```python
from build123d import *

# Parameters (mm, degrees)
BOSS_EXTRUDE3_DEPTH        = 10
SKETCH4_R                  = 1.5
BOSS_EXTRUDE4_DEPTH        = 5
RIB6_REACH                 = 158.985
SKETCH5_WALL_W             = 329.861950248
SKETCH5_WALL_H             = 2.5
CHAMFER2_SIZE              = 1
LPATTERN4_COUNT            = 2
LPATTERN4_PITCH            = 75
LPATTERN4_COPY_1_REACH     = 158.985
LPATTERN4_COPY_1_SKETCH_W  = 329.861950248
LPATTERN4_COPY_1_SKETCH_H  = 2.5
CHAMFER2_OF_LPATTERN4_SIZE = 1
CHAMFER3_SIZE              = 9
SKETCH8_R                  = 2.05
CUT_EXTRUDE1_DEPTH         = 4
SKETCH9_R                  = 1.6
CUT_EXTRUDE2_DEPTH         = 5


with BuildPart() as part:
    # Sketch2 → Boss-Extrude3 (new body)
    with BuildSketch(Plane(origin=(0, 0, 0), x_dir=(1, 0, 0), z_dir=(0, 1, 0))):
        with BuildLine():
            Line((-138.973021921, 39.179223473), (-139.052157616, 4.179312937))
            Line((-139.052157616, 4.179312937), (73.947297933, 3.697715709))
            Line((73.947297933, 3.697715709), (74.026978079, 38.697625014))
            Line((74.026978079, 38.697625014), (67.526578048, 38.712322585))
            Line((67.526578048, 38.712322585), (67.51414235, 33.212297518))
            Line((67.51414235, 33.212297518), (58.599731895, 33.232453229))
            ThreePointArc((58.599731895, 33.232453229), (42.488076808, 21.768891824), (26.428425, 33.305193378))
            Line((26.428425, 33.305193378), (17.51414235, 33.3253488))
            Line((17.51414235, 33.3253488), (17.526578048, 38.825373866))
            Line((17.526578048, 38.825373866), (-7.473230244, 38.881899074))
            Line((-7.473230244, 38.881899074), (-7.485665941, 33.381874007))
            Line((-7.485665941, 33.381874007), (-16.400076396, 33.402029717))
            ThreePointArc((-16.400076396, 33.402029717), (-32.511731484, 21.938468313), (-48.571383292, 33.474769867))
            Line((-48.571383292, 33.474769867), (-57.485665941, 33.494925288))
            Line((-57.485665941, 33.494925288), (-57.473230244, 38.994950355))
            Line((-57.473230244, 38.994950355), (-82.473038536, 39.051475562))
            Line((-82.473038536, 39.051475562), (-82.485474233, 33.551450496))
            Line((-82.485474233, 33.551450496), (-91.399884688, 33.571606206))
            ThreePointArc((-91.399884688, 33.571606206), (-107.511539776, 22.108044802), (-123.571191584, 33.644346356))
            Line((-123.571191584, 33.644346356), (-132.485474233, 33.664501777))
            Line((-132.485474233, 33.664501777), (-132.473038536, 39.164526844))
            Line((-132.473038536, 39.164526844), (-138.973021921, 39.179223473))
        make_face()
    extrude(amount=BOSS_EXTRUDE3_DEPTH)

    # Sketch4 → Boss-Extrude4 (add)
    with BuildSketch(Plane(origin=(0.087874316, 0, -38.864803222), x_dir=(-0.99999744389135, 0, -0.002261019850970016), z_dir=(0.002261019850970016, 0, -0.99999744389135))):
        Polygon((62.56118779, -12), (57.561251693, 0), (82.561123887, 0), (77.56118779, -12), align=None)
        with Locations((70.06118779, -8.5)):
            Circle(SKETCH4_R, mode=Mode.SUBTRACT)
    boss_extrude4 = extrude(amount=-BOSS_EXTRUDE4_DEPTH)

    # Sketch5 wall → Rib6 (add, up to next)
    with BuildSketch(Plane(origin=(-77.492333887, -6, -30.540192335), x_dir=(-0.001139262394, 0.863778900906, 0.503869737562), z_dir=(-0.001953021242, -0.503871025511, 0.863776692993)), mode=Mode.PRIVATE) as rib6_sk1:
        with Locations((0, -1.25)):
            Rectangle(SKETCH5_WALL_W, SKETCH5_WALL_H)
    rib6_tool1 = extrude(rib6_sk1.sketch, amount=-RIB6_REACH, mode=Mode.PRIVATE) - part.part
    rib6 = rib6_tool1.solids().sort_by_distance((-77.492333887, -6, -30.540192335))[0]
    add(rib6)

    # Mirror2: Rib6 across plane
    add(rib6.mirror(Plane(origin=(-70.061008706, 0, -0.158409736), x_dir=(-0.0022610198509701073, 0, 0.99999744389135), z_dir=(0.99999744389135, 0, 0.002261019850970107))))

    # Chamfer2
    chamfer2_edges = [part.edges().sort_by_distance(p)[0] for p in [
        (-68.484443323, -8.5, -34.01983421),
    ]]
    chamfer(chamfer2_edges, length=CHAMFER2_SIZE)

    # LPattern4: Boss-Extrude4, Rib6 ×2
    with Locations(*[Vector(0.9999974438913499, 0, 0.002261019850970079) * (i * LPATTERN4_PITCH) for i in range(1, LPATTERN4_COUNT)]):
        add(boss_extrude4)
        add(rib6)

    # LPattern4 copy 1 sketch → LPattern4 copy 1 (add, up to next)
    with BuildSketch(Plane(origin=(12.507436062, -6, -30.336700548), x_dir=(-0.0011392623880184954, 0.863778900906, 0.5038697375620136), z_dir=(-0.0019530212415939509, -0.503871025511, 0.863776692993001)), mode=Mode.PRIVATE) as lpattern4_copy_1_sk1:
        with Locations((0, 1.25)):
            Rectangle(LPATTERN4_COPY_1_SKETCH_W, LPATTERN4_COPY_1_SKETCH_H)
    lpattern4_copy_1_tool1 = extrude(lpattern4_copy_1_sk1.sketch, amount=-LPATTERN4_COPY_1_REACH, mode=Mode.PRIVATE) - part.part
    add(lpattern4_copy_1_tool1.solids().sort_by_distance((12.507436062, -6, -30.336700548))[0])

    # Chamfer2 of LPattern4
    chamfer2_of_lpattern4_edges = [part.edges().sort_by_distance(p)[0] for p in [
        (6.515364969, -8.5, -33.850257721),
    ]]
    chamfer(chamfer2_of_lpattern4_edges, length=CHAMFER2_OF_LPATTERN4_SIZE)

    # Chamfer3
    chamfer3_edges = [part.edges().sort_by_distance(p)[0] for p in [
        (-32.552429841, 0, -3.938514323),
    ]]
    chamfer(chamfer3_edges, length=CHAMFER3_SIZE)

    # Sketch8 → Cut-Extrude1 (cut)
    with BuildSketch(Plane(origin=(0, 10, 0), x_dir=(1, 0, 0), z_dir=(0, 1, 0))):
        with Locations(Location((-129.018242433, 19.156613217, 0), (0, 0, 270))):
            Circle(SKETCH8_R)
    cut_extrude1 = extrude(amount=-CUT_EXTRUDE1_DEPTH, mode=Mode.SUBTRACT)

    # Sketch9 → Cut-Extrude2 (cut)
    with BuildSketch(Plane(origin=(0, 6, 0), x_dir=(1, 0, 0), z_dir=(0, 1, 0))):
        with Locations(Location((-129.018242433, 19.156613217, 0), (0, 0, 270))):
            Circle(SKETCH9_R)
    cut_extrude2 = extrude(amount=-CUT_EXTRUDE2_DEPTH, mode=Mode.SUBTRACT)

    # Mirror4: Cut-Extrude1, Cut-Extrude2 across plane
    add(cut_extrude1.mirror(Plane(origin=(-32.561168463, 0, -0.073621636), x_dir=(-0.002261019850969509, 0, 0.99999744389135), z_dir=(-0.99999744389135, 0, -0.0022610198509695084))), mode=Mode.SUBTRACT)
    add(cut_extrude2.mirror(Plane(origin=(-32.561168463, 0, -0.073621636), x_dir=(-0.002261019850969509, 0, 0.99999744389135), z_dir=(-0.99999744389135, 0, -0.0022610198509695084))), mode=Mode.SUBTRACT)


solid = part.part
```
Check sheet for the modelled part. Datum: model origin and axes. Units: mm. A direction names the side the tool comes from. Round coordinates to 2 decimals unless told otherwise and drop trailing zeros. Order: outer loops, then holes, each group sorted by start corner. A loop starts at its lowest first (then second) coordinate and runs counter-clockwise, first axis right, second up.
1) Section check B-B (y = 3). Record the boundary of the cut face in (x, z).
2) Go/stop test with flat-tipped pins: pin 1 Ø2 at (x, z) = (-8.5, -26) entering from -Y; pin 2 Ø12 at (x, y) = (11.5, 6) entering from -Z; pin 3 Ø2 at (x, z) = (63, -18.5) entering from +Y. Record where each tip stops, or that it passes through.
3) Section check A-A (z = -29). Give the number of separate pieces and of enclosed holes in the cut face, and give its area (3 significant figures).
4) Section check C-C (x = -104). Record the boundary of the cut face in (y, z).
5) Scan lines: line 1 (X direction, y = -1.25, z = -28.5); line 2 (X direction, y = 0.75, z = -35); line 3 (Z direction, x = -53, y = 0.25). Record each from-to range of solid material in increasing order.
6) Section check D-D (x = -39). Record the boundary of the cut face in (y, z).
7) Tool access check on faces 1 (the cylindrical face through (-107.22, 4.93, -22.11)), 2 (the flat face through (-34, 0, -20)). Record the directions out of +Z, -Z, +X, -X, +Y, -Y that give a thin tool (end or side, any length) a straight path to the whole face; none if there is none.
Result:
1. outline: (-139.04, -10.18) - (-138.97, -39.18) - (-132.47, -39.16) - (-132.49, -33.66) - (-123.57, -33.64) arc R17 cw to (-91.4, -33.57) - (-82.49, -33.55) - (-82.47, -39.05) - (-57.47, -38.99) - (-57.49, -33.49) - (-48.57, -33.47) arc R17 cw to (-16.4, -33.4) - (-7.49, -33.38) - (-7.47, -38.88) - (17.53, -38.83) - (17.51, -33.33) - (26.43, -33.31) arc R17 cw to (58.6, -33.23) - (67.51, -33.21) - (67.53, -38.71) - (74.03, -38.7) - (73.96, -9.7) - close; hole circle Ø3.2 at (-129.02, -19.16); hole circle Ø3.2 at (63.98, -18.72)
2. pin 1: stops at y = 0
2. pin 2: stops at z = -38.85
2. pin 3: stops at y = 6
3. separate pieces: 4
3. enclosed holes: 0
3. area: 1,340 mm2
4. outline: (0, -22.47) - (10, -22.47) - (10, -4.1) - (9, -4.1) - (0, -13.1) - close
5. line 1: x = -77.5 to -75, -65 to -62.5, -2.5 to 0, 10 to 12.5
5. line 2: x = -138.98 to -132.48, -82.48 to -57.48, -7.48 to 17.52, 67.52 to 74.02
5. line 3: z = -33.48 to -12.73
6. outline: (0, -23.24) - (10, -23.24) - (10, -3.95) - (9, -3.95) - (0, -12.95) - close
7. face 1: -Z, +Y, -Y
7. face 2: +Z, -Y
